Check sheet for the drawn part. Datum: minimum x, y, z corner. Units: mm. A direction names the side the tool comes from. Give positions to 0.01 mm unless a question says otherwise; leave off trailing zeros. Write each loop counter-clockwise with the first axis right and the second up, starting at its lowest first coordinate (ties: lowest second). Pieces come first, ordered by that corner, then holes.
(1) Cross-section at B-B (x = 72). Record the boundary of the cut face in (y, z) (1 decimal), and give its area (3 significant figures).
(2) Tool access check on the marked faces 4, 5 and 6. Record the directions out of +Z, -Z, +X, -X, +Y, -Y that give a thin tool (end or side, any length) a straight path to the whole face; none if there is none.
(3) Thickness scan on line 1 along X through (y, z) = (13.5, 20); line 2 along Z through (x, y) = (52, 2) (1 decimal); line 3 along X through (y, z) = (11.5, 16) (1 decimal). Record the ranges inside material, lowest first.
(4) Cross-section at A-A (z = 20). Record the boundary of the cut face in (x, y), and give its area (3 significant figures).
(5) Cross-section at D-D (x = 27.5). Record the boundary of the cut face in (y, z).
(6) Mould release check, pull along Z, two halves, no side actions. Record for the marked faces 1, 2 and 3: +Z half, -Z half, draft (parallel to the pull), parting line (faces both ways), or undercut.
(7) Depth check by flat-ended pin: P1, Ø6, axis at y = 12.5, z = 65, coming from the -X side; P2, Ø18, axis at x = 60.28, z = 20, coming from the -Y side; P3, Ø6, axis at x = 56, y = 10, coming from the -Z side; P4, Ø4, axis at x = 23, y = 10.5, coming from the -Z side. Enter the tip coordinate at first touch or a pass-through.
(8) Cross-section at C-C (z = 96.5). Record the boundary of the cut face in (x, y) (1 decimal), and give its area (3 significant figures).
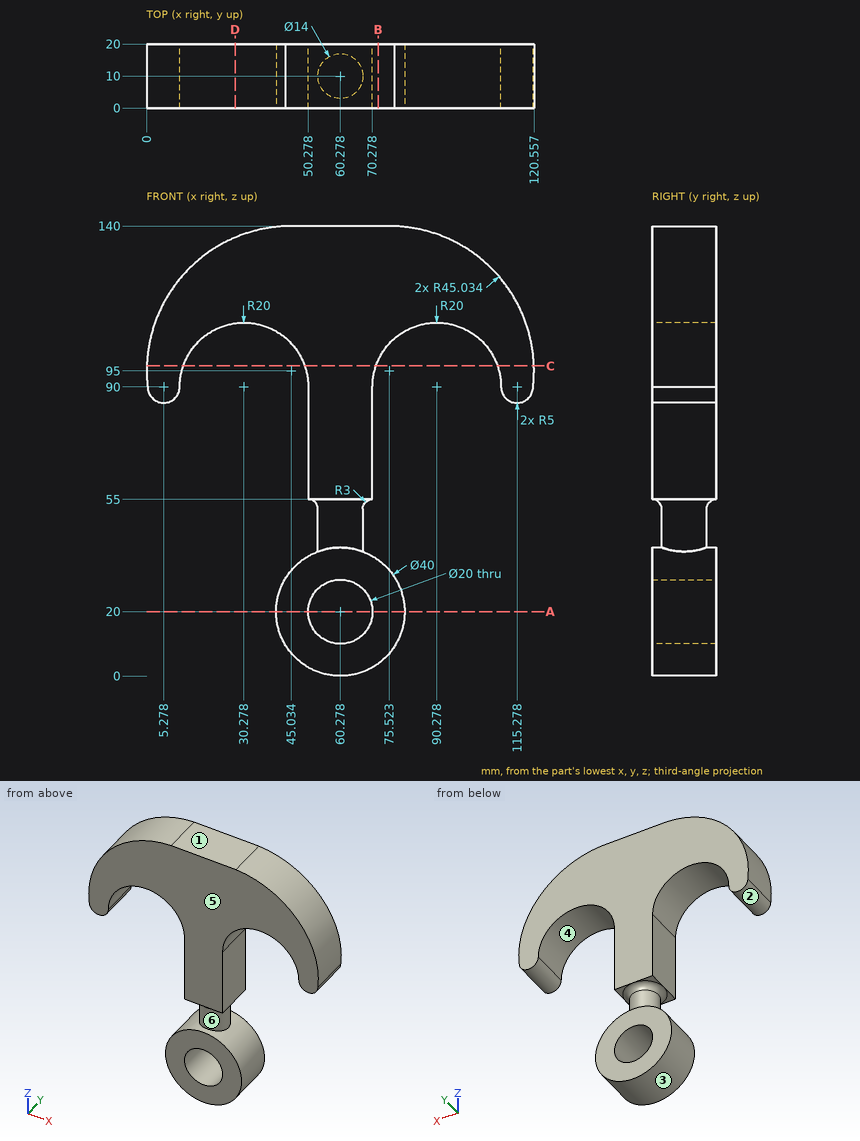
Reply:
1. outline: (0, 3.8) - (20, 3.8) - (20, 36.2) - (0, 36.2) - close; (0, 98.1) - (20, 98.1) - (20, 140) - (0, 140) - close
1. area: 1,490 mm2
2. face 4: +Y, -Y
2. face 5: +Z, -Z, +X, -X, -Y
2. face 6: none
3. line 1: x = 40.28 to 50.28, 70.28 to 80.28
3. line 2: z = 1.8 to 14.4, 25.6 to 38.2, 55 to 140
3. line 3: x = 40.7 to 51.1, 69.4 to 79.9
4. outline: (40.28, 0) - (50.28, 0) - (50.28, 20) - (40.28, 20) - close; (70.28, 0) - (80.28, 0) - (80.28, 20) - (70.28, 20) - close
4. area: 400 mm2
5. outline: (0, 109.81) - (20, 109.81) - (20, 136.48) - (0, 136.48) - close
6. face 1: +Z half
6. face 2: -Z half
6. face 3: undercut
7. P1: stops at x = 50.28
7. P2: passes through
7. P3: stops at z = 0.04
7. P4: stops at z = 107.72
8. outline: (0, 0) - (11.4, 0) - (11.4, 20) - (0, 20) - close; (49.2, 0) - (71.4, 0) - (71.4, 20) - (49.2, 20) - close; (109.2, 0) - (120.5, 0) - (120.5, 20) - (109.2, 20) - close
8. area: 897 mm2
